Part model, mm, in its own coordinate system. Face numbers are marked on the shaded views. A direction names the side the tool comes from. Coordinates: 2 decimals unless noted, no trailing zeros. Loops run counter-clockwise (first coordinate to the right, second up) from the corner with the lowest first, then second, coordinate; pieces in that order, holes last. Notation, with made-up numbers: (-33, 3) - (-18, 3) arc R8 cw to (-18, 9) - close; hole circle Ø6 at (-29, 68). An arc over 180 degrees is marked (long way). Answer as CSV lines item,"result".
from build123d import *

# Parameters (mm, degrees)
PAD034_DEPTH    = 19.05
SKETCH070_R     = 1.778
POCKET004_DEPTH = 15.876
SKETCH071_R     = 2.794
POCKET005_DEPTH = 3.048


with BuildPart() as part:
    # Sketch069 → Pad034 (new body)
    with BuildSketch(Plane.YZ):
        with BuildLine():
            Line((-19.05, -7.9375), (-19.05, 7.9375))
            Line((-19.05, 7.9375), (19.05, 7.9375))
            Line((19.05, 7.9375), (19.05, -7.9375))
            Line((19.05, -7.9375), (12.364569, -7.9375))
            ThreePointArc((12.364569, -7.9375), (0, 3.9295), (-12.364569, -7.9375))
            Line((-12.364569, -7.9375), (-19.05, -7.9375))
        make_face()
    extrude(amount=PAD034_DEPTH)

    # Sketch070 (on Face2 of Pad034) → Pocket004 (cut, through all)
    with BuildSketch(Plane(origin=(0, 0, 7.9375), x_dir=(0, -1, 0), z_dir=(0, 0, 1))):
        with Locations((15.875, 15.875)):
            Circle(SKETCH070_R)
        with Locations((15.875, 3.175)):
            Circle(SKETCH070_R)
        with Locations((-15.875, 15.875)):
            Circle(SKETCH070_R)
        with Locations((-15.875, 3.175)):
            Circle(SKETCH070_R)
    extrude(amount=-POCKET004_DEPTH, mode=Mode.SUBTRACT)

    # Sketch071 (on Face2 of Pad034) → Pocket005 (cut)
    with BuildSketch(Plane(origin=(0, 0, 7.9375), x_dir=(0, -1, 0), z_dir=(0, 0, 1))):
        with Locations((15.875, 15.875)):
            Circle(SKETCH071_R)
        with Locations((15.875, 3.175)):
            Circle(SKETCH071_R)
        with Locations((-15.875, 15.875)):
            Circle(SKETCH071_R)
        with Locations((-15.875, 3.175)):
            Circle(SKETCH071_R)
    extrude(amount=-POCKET005_DEPTH, mode=Mode.SUBTRACT)


with BuildPart() as part_1:
    # Body027 placement: moved
    add(part.part.moved(Location((-17.78, 40.132, 16.256))))


solid = part_1.part
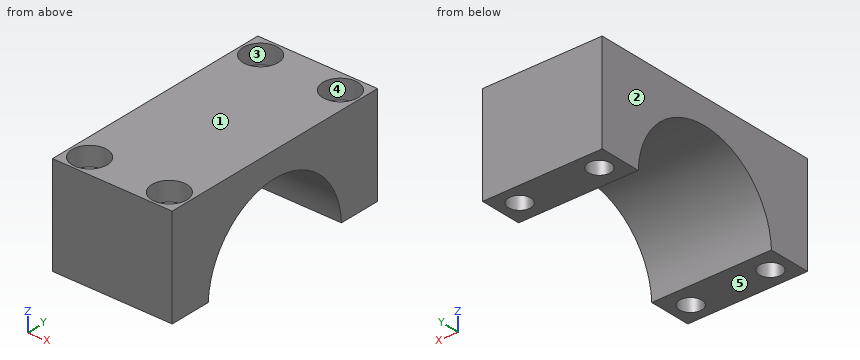
Q1. Flat gauge pins, fed straight in: pin 1 (4 mm diameter, centred on x = -1.905, y = 56.007, fed in from +Z); pin 2 (10 mm diameter, centred on x = -12.5, y = 38.5, fed in from -Z). Where does each tip first touch, or does it go through?
Results:
pin 1,"stops at z = 21.15"
pin 2,"stops at z = 18.26"
Q2. Two-plate mould, pull along X, no slides. Class the marked faces 1, 2 and 3: released by +X, released by -X, zero draft, split by the parting line, or undercut.
Results:
face 1,"zero draft"
face 2,"released by -X"
face 3,"undercut"
Q3. Which spindle directions (+Z, -Z, +X, -X, +Y, -Y) get a long thin tool onto all of the face, cutting with end or side? Do the marked faces 4 and 5. Say none if no direction does.
Results:
face 4,"+Z"
face 5,"-Z, +X, -X, +Y, -Y"
Q4. Wall check: L1, parallel to Y at x = -2, z = 22.5; L2, parallel to Y at x = -3.5, z = 14.25; L3, parallel to Y at x = -3.5, z = 11.5. Give the ranges that are in metal, low to high.
Results:
L1,"y = 21.08 to 21.46, 27.05 to 53.21, 58.8 to 59.18"
L2,"y = 21.08 to 23.47, 25.04 to 29.56, 50.7 to 55.22, 56.79 to 59.18"
L3,"y = 21.08 to 23.47, 25.04 to 28.32, 51.94 to 55.22, 56.79 to 59.18"
Q5. Saw through at C-C (z = 17). Give the cut face in (x, y) (3 decimals), then the cut area to 3 significant figures.
Results:
outline,"(-17.78, 21.082) - (1.27, 21.082) - (1.27, 31.844) - (-17.78, 31.844) - close; (-17.78, 48.42) - (1.27, 48.42) - (1.27, 59.182) - (-17.78, 59.182) - close; hole circle Ø3.556 at (-14.605, 24.257); hole circle Ø3.556 at (-14.605, 56.007); hole circle Ø3.556 at (-1.905, 24.257); hole circle Ø3.556 at (-1.905, 56.007)"
area,"370 mm^2"
Q6. Saw through at B-B (x = -1.25). Count the separate pieces of the cut face and the enclosed holes in it, then the cut area to 3 significant figures.
Results:
separate pieces,"3"
enclosed holes,"0"
area,"259 mm^2"
Q7. Saw through at A-A (z = 19). Give the cut face in (x, y) (3 decimals), then the cut area to 3 significant figures.
Results:
outline,"(-17.78, 21.082) - (1.27, 21.082) - (1.27, 34.847) - (-17.78, 34.847) - close; (-17.78, 45.417) - (1.27, 45.417) - (1.27, 59.182) - (-17.78, 59.182) - close; hole circle Ø3.556 at (-14.605, 24.257); hole circle Ø3.556 at (-14.605, 56.007); hole circle Ø3.556 at (-1.905, 24.257); hole circle Ø3.556 at (-1.905, 56.007)"
area,"485 mm^2"
